```python
from build123d import *

# Parameters (mm, degrees)
F1_DEPTH = 25.4
F4_DEPTH = 12.7
F2_R     = 6.35
F5_DEPTH = 25.4


# Not quite as in the source:
# - ends of sketch curves that miss each other by under 0.0002 mm in the source are joined


with BuildPart() as f1:
    # F0 (on Front) → F1 (new body)
    with BuildSketch(Plane.XZ):
        Polygon((-46.4223937518, 20.1214007731), (-71.8223937518, 20.1214007731), (-71.8223937518, -17.9785992269), (-1.9723937518, -17.9785992269), (-1.9723937518, -5.2785992269), (-46.4223937518, -5.2785992269), align=None)
    extrude(amount=F1_DEPTH)

    # F3 (on face) → F4 (cut)
    with BuildSketch(Plane.XY.offset(-5.2785992269)):
        with BuildLine():
            ThreePointArc((-8.3223937518, -12.6999999235), (-10.1822656913, -8.2098718629), (-14.6723937518, -6.3499999235))
            ThreePointArc((-14.6723937518, -6.3499999235), (-21.0223937518, -12.6999999235), (-14.6723937518, -19.0499999235))
            ThreePointArc((-14.6723937518, -19.0499999235), (-10.1822656913, -17.190127984), (-8.3223937518, -12.6999999235))
        make_face()
        with BuildLine():
            ThreePointArc((-33.7223937518, -6.3499998086), (-29.2322656913, -8.2098717481), (-27.3723937518, -12.6999998086))
            ThreePointArc((-27.3723937518, -12.6999998086), (-29.2322656913, -17.1901278692), (-33.7223937518, -19.0499998086))
            Line((-33.7223937518, -19.0499998086), (-14.6723937518, -19.0499998086))
            ThreePointArc((-14.6723937518, -19.0499998086), (-21.0223937518, -12.6999999235), (-14.6723937518, -6.3499999235))
            Line((-14.6723937518, -6.3499999235), (-33.7223937518, -6.3499998086))
        make_face()
        with BuildLine():
            ThreePointArc((-33.7223937518, -19.0499998086), (-29.2322656913, -17.1901278692), (-27.3723937518, -12.6999998086))
            ThreePointArc((-27.3723937518, -12.6999998086), (-29.2322656913, -8.2098717481), (-33.7223937518, -6.3499998086))
            ThreePointArc((-33.7223937518, -6.3499998086), (-40.0723937518, -12.6999998086), (-33.7223937518, -19.0499998086))
        make_face()
    extrude(amount=-F4_DEPTH, mode=Mode.SUBTRACT)

    # F2 (on face) → F5 (cut)
    with BuildSketch(Plane.XZ.offset(25.4)):
        with Locations((-59.1223937518, 7.4214007731)):
            Circle(F2_R)
        with BuildLine():
            ThreePointArc((-71.8223937518, 7.4214007731), (-59.1223937518, 20.1043120223), (-46.4223937518, 7.4214007731))
            Line((-46.4223937518, 7.4214007731), (-46.4223937518, 20.1214007731))
            Line((-46.4223937518, 20.1214007731), (-71.8223937518, 20.1214007731))
            Line((-71.8223937518, 20.1214007731), (-71.8223937518, 7.4214007731))
        make_face()
    extrude(amount=-F5_DEPTH, mode=Mode.SUBTRACT)


solid = f1.part
```
The listing builds one solid part. Answer for the finished solid, in the listing's coordinates (mm). A direction names the side the tool comes from. Round coordinates to 2 decimals unless told otherwise and drop trailing zeros. Write each loop counter-clockwise with the first axis right and the second up, starting at its lowest first coordinate (ties: lowest second). Pieces come first, ordered by that corner, then holes. Notation, with made-up numbers: (10.25, 18.25) -> (68.25, 18.25) arc R13 cw to (68.25, 33.25) -> close; hole circle Ø1 at (81.5, 44). An arc over 180 degrees is marked (long way). Answer as a JSON object with one key per item and string values. Group by question number.
Q1. Section D-D (z = -8.5) is taken. Write down the section's boundary in (x, y), plus the area to 3 significant figures.
Q2. Each of these flat-tipped pins is pushed along its axis until it touches: pin 1 Ø4 at (x, y) = (-61.5, -8.5) entering from +Z; pin 2 Ø6 at (x, y) = (-16, -18.5) entering from +Z; pin 3 Ø10 at (x, z) = (-59.12, 7.42) entering from -Y; pin 4 Ø6.5 at (y, z) = (-16.5, 4) entering from +X. Where does it stop, or does it pass through?
Q3. Determine the mould class of faces 4 (the face through (-24, -4, -5.279)), 5 (the face through (-24, -19.05, -12)), 6 (the face through (-45, -25.4, -7)) for opening direction Y: pulls with the +Y half, pulls with the -Y half, needs draft (parallel to the pull), parting line crosses it, or undercut.
Q4. Section A-A (x = -26) is taken. Write down the section's boundary in (y, z).
Q5. Section C-C (z = 12.5) is taken. Write down the section's boundary in (x, y), plus the area to 3 significant figures.
Q6. Straight lines are drawn through the part: line 1 along Y through (x, z) = (-15.5, -14.5); line 2 along Z through (x, y) = (-59.5, -23.25); line 3 along Z through (x, y) = (-15.5, -24). For each, find the intervals that lie inside material, in ascending order.
Q7. Section B-B (y = -4) is taken. Write down the section's boundary in (x, z).
Q8. Which of the six approach directions +Z, -Z, +X, -X, +Y, -Y give full straight-line access (tool end or side, diameter ignored) to faces 1 (the face through (-46.422, -13, 1)), 2 (the face through (-1.972, -13, -12)), 3 (the face through (-24, -6.35, -12))?
Check values:
{
 "1": {"outline": "(-71.82, -25.4) -> (-1.97, -25.4) -> (-1.97, 0) -> (-71.82, 0) -> close; hole (-33.72, -19.05) -> (-14.67, -19.05) arc R6.35 ccw to (-14.67, -6.35) -> (-33.72, -6.35) arc R6.35 ccw to start", "area": "1,410 mm^2"},
 "2": {"pin 1": "z = 20.1", "pin 2": "z = -5.28", "pin 3": "through", "pin 4": "x = -46.42"},
 "3": {"face 4": "needs draft", "face 5": "undercut", "face 6": "pulls with the -Y half"},
 "4": {"outline": "(-25.4, -17.98) -> (-19.05, -17.98) -> (-19.05, -5.28) -> (-25.4, -5.28) -> close; (-6.35, -17.98) -> (0, -17.98) -> (0, -5.28) -> (-6.35, -5.28) -> close"},
 "5": {"outline": "(-70.76, -25.4) -> (-62.93, -25.4) -> (-62.93, 0) -> (-70.76, 0) -> close; (-55.31, -25.4) -> (-47.49, -25.4) -> (-47.49, 0) -> (-55.31, 0) -> close", "area": "397 mm^2"},
 "6": {"line 1": "-25.4 to -19.05, -6.35 to 0", "line 2": "-17.98 to 1.08, 13.76 to 20.1", "line 3": "-17.98 to -5.28"},
 "7": {"outline": "(-71.82, -17.98) -> (-1.97, -17.98) -> (-1.97, -5.28) -> (-46.42, -5.28) -> (-46.42, 7.42) arc R12.7 ccw to (-71.82, 7.42) -> close; hole circle Ø12.7 at (-59.12, 7.42)"},
 "8": {"face 1": "+Z, +X, +Y, -Y", "face 2": "+Z, -Z, +X, +Y, -Y", "face 3": "+Z, -Z"}
}
